The model under review builds one solid part; all positions refer to its coordinate system, in mm. A direction names the side the tool comes from. Give positions to 0.01 mm unless a question says otherwise; leave off trailing zeros. Order: outer loops, then holes, each group sorted by start corner. A loop starts at its lowest first (then second) coordinate and runs counter-clockwise, first axis right, second up. Notation, with made-up numbers: (1.25, 32.5) - (19.25, 32.5) arc R20 cw to (19.25, 38.5) - close; hole circle Ø6 at (-29, -28.5). An arc over 180 degrees is marked (long way). Use CSV: the item, a comma, the result in double quotes. Start each with the question number.
1. Machinability: for faces 4 (the flat face through (-1, 1, 50)), 5 (the flat face through (-1, 51, 0)), which of the approach directions +Z, -Z, +X, -X, +Y, -Y give a long, thin tool a straight path to every point of the face, cutting with its end or side? Answer none if there is none.
2. Take a section at B-B, the plane x = 0. State the section outline as (y, z) points, then the cut area to 3 significant figures.
3. Draft analysis for pull direction X (two halves, no side actions). For faces 1 (the flat face through (-1, 1, -50)), 2 (the cylindrical face through (-8.13, -76.61, 24.65)), 3 (the flat face through (-100, -1, -1)), state which applies: released by +X, released by -X, zero draft, split by the parting line, or undercut.
4. Take a section at A-A, the plane y = 50. State the section outline as (x, z) points.
5. To check wall thickness, follow line 1 (Y direction, x = 0, z = 27); line 2 (Y direction, x = -26, z = 11); line 3 (X direction, y = -6, z = 33). State the ranges of each line that lie inside material, in increasing order. Write a range as [from, to].
6. For pin 1 (22.5 mm diameter, centred on x = -13, y = -45, fed in from +Z), flat-tipped, find the tip position at first contact; note if it passes through.
7. Take a section at C-C, the plane z = 14. State the section outline as (x, y) points.
8. Take a section at D-D, the plane y = -73. State the section outline as (x, z) points, then the cut area to 3 significant figures.
```python
from build123d import *

# Parameters (mm, degrees)
F2_W     = 200
F2_H     = 200
F2_R     = 37.5
F3_DEPTH = 50
F4_DEPTH = 50


with BuildPart() as f3:
    # F2 (on Top) → F3 (new body)
    with BuildSketch(Plane.XY):
        Rectangle(F2_W, F2_H)
        with Locations((0, -40)):
            Circle(F2_R, mode=Mode.SUBTRACT)
        with Locations((0, 50)):
            Circle(F2_R, mode=Mode.SUBTRACT)
        with Locations((0, -40)):
            Circle(F2_R)
        with Locations((0, 50)):
            Circle(F2_R)
    extrude(amount=-F3_DEPTH)

    # F2 (on Top) → F4 (join)
    with BuildSketch(Plane.XY):
        Rectangle(F2_W, F2_H)
        with Locations((0, -40)):
            Circle(F2_R, mode=Mode.SUBTRACT)
        with Locations((0, 50)):
            Circle(F2_R, mode=Mode.SUBTRACT)
    extrude(amount=F4_DEPTH)


solid = f3.part
```
Determined:
1,face 4,"+Z, +X, -X, +Y, -Y"
1,face 5,"+Z"
2,outline,"(-100, -50) - (100, -50) - (100, 50) - (87.5, 50) - (87.5, 0) - (12.5, 0) - (12.5, 50) - (-2.5, 50) - (-2.5, 0) - (-77.5, 0) - (-77.5, 50) - (-100, 50) - close"
2,area,"12,500 mm²"
3,face 1,"zero draft"
3,face 2,"undercut"
3,face 3,"released by -X"
4,outline,"(-100, -50) - (100, -50) - (100, 50) - (37.5, 50) - (37.5, 0) - (-37.5, 0) - (-37.5, 50) - (-100, 50) - close"
5,line 1,"y = [-100, -77.5], [-2.5, 12.5], [87.5, 100]"
5,line 2,"y = [-100, -67.02], [-12.98, 22.98], [77.02, 100]"
5,line 3,"x = [-100, -15.82], [15.82, 100]"
6,pin 1,"stops at z = 0"
7,outline,"(-100, -100) - (100, -100) - (100, 100) - (-100, 100) - close; hole circle Ø75 at (0, -40); hole circle Ø75 at (0, 50)"
8,outline,"(-100, -50) - (100, -50) - (100, 50) - (17.81, 50) - (17.81, 0) - (-17.81, 0) - (-17.81, 50) - (-100, 50) - close"
8,area,"18,200 mm²"
